from build123d import *

# Parameters (mm, degrees)
BOSS_EXTRUDE1_DEPTH      = 22
BOSS_EXTRUDE1_DEPTH_BACK = 22
SKETCH2_W                = 38
SKETCH2_H                = 20
CUT_EXTRUDE1_DEPTH       = 105.423416914
SKETCH3_W                = 7
SKETCH3_H                = 44
BOSS_EXTRUDE2_DEPTH      = 65.5
SKETCH23_R               = 5
SKETCH23_R_2             = 1.2
CUT_EXTRUDE2_DEPTH       = 111.605436123
SKETCH24_W               = 28.5
SKETCH24_H               = 34
CUT_EXTRUDE3_DEPTH       = 90.954502389
SKETCH26_R               = 1.2
SKETCH26_R_2             = 5
SKETCH26_R_3             = 1.45
CUT_EXTRUDE6_DEPTH       = 107.330263801
SKETCH27_W               = 29.7
SKETCH27_H               = 35.2
CUT_EXTRUDE8_DEPTH       = 73.137455597
SKETCH29_W               = 7
SKETCH29_H               = 30
CUT_EXTRUDE10_DEPTH      = 74.468530678
CHAMFER2_SIZE            = 5


with BuildPart() as part:
    # Sketch1 → Boss-Extrude1 (new, two sides: drawn at the far end of the back side and taken through both)
    with BuildSketch(Plane.XY.offset(-BOSS_EXTRUDE1_DEPTH_BACK)):
        with BuildLine():
            Line((10.25, -60), (10.25, 0))
            ThreePointArc((10.25, 0), (0, -10.25), (-10.25, 0))
            Line((-10.25, 0), (-10.25, -60))
            Line((-10.25, -60), (-10.25, -100))
            Line((-10.25, -100), (10.25, -100))
            Line((10.25, -100), (10.25, -60))
        make_face()
        with BuildLine():
            Line((10.25, 0), (9.2, 0))
            ThreePointArc((9.2, 0), (8.816088231, -0.879772698), (7.91, -1.196620241))
            ThreePointArc((7.91, -1.196620241), (5.656854249, -5.656854249), (1.196620241, -7.91))
            ThreePointArc((1.196620241, -7.91), (1.199154762, -7.954968281), (1.2, -8))
            ThreePointArc((1.2, -8), (-0.045031719, -9.199154762), (-1.196620241, -7.91))
            ThreePointArc((-1.196620241, -7.91), (-5.656854249, -5.656854249), (-7.91, -1.196620241))
            ThreePointArc((-7.91, -1.196620241), (-8.816088231, -0.879772698), (-9.2, 0))
            Line((-9.2, 0), (-10.25, 0))
            ThreePointArc((-10.25, 0), (0, -10.25), (10.25, 0))
        make_face()
        with BuildLine():
            ThreePointArc((7.91, -1.196620241), (7.120227302, -0.816088231), (6.8, 0))
            Line((6.8, 0), (4.2, 0))
            ThreePointArc((4.2, 0), (0, -4.2), (-4.2, 0))
            Line((-4.2, 0), (-6.8, 0))
            ThreePointArc((-6.8, 0), (-7.120227302, -0.816088231), (-7.91, -1.196620241))
            ThreePointArc((-7.91, -1.196620241), (-5.656854249, -5.656854249), (-1.196620241, -7.91))
            ThreePointArc((-1.196620241, -7.91), (0, -6.8), (1.196620241, -7.91))
            ThreePointArc((1.196620241, -7.91), (5.656854249, -5.656854249), (7.91, -1.196620241))
        make_face()
        with BuildLine():
            Line((4.2, 0), (6.8, 0))
            ThreePointArc((6.8, 0), (7.120227302, 0.816088231), (7.91, 1.196620241))
            ThreePointArc((7.91, 1.196620241), (5.656854249, 5.656854249), (1.196620241, 7.91))
            ThreePointArc((1.196620241, 7.91), (0, 6.8), (-1.196620241, 7.91))
            ThreePointArc((-1.196620241, 7.91), (-5.656854249, 5.656854249), (-7.91, 1.196620241))
            ThreePointArc((-7.91, 1.196620241), (-7.120227302, 0.816088231), (-6.8, 0))
            Line((-6.8, 0), (-4.2, 0))
            ThreePointArc((-4.2, 0), (0, 4.2), (4.2, 0))
        make_face()
        with BuildLine():
            ThreePointArc((7.91, 1.196620241), (8.816088231, 0.879772698), (9.2, 0))
            Line((9.2, 0), (10.25, 0))
            ThreePointArc((10.25, 0), (0, 10.25), (-10.25, 0))
            Line((-10.25, 0), (-9.2, 0))
            ThreePointArc((-9.2, 0), (-8.816088231, 0.879772698), (-7.91, 1.196620241))
            ThreePointArc((-7.91, 1.196620241), (-5.656854249, 5.656854249), (-1.196620241, 7.91))
            ThreePointArc((-1.196620241, 7.91), (-0.045031719, 9.199154762), (1.2, 8))
            ThreePointArc((1.2, 8), (1.199154762, 7.954968281), (1.196620241, 7.91))
            ThreePointArc((1.196620241, 7.91), (5.656854249, 5.656854249), (7.91, 1.196620241))
        make_face()
    extrude(amount=BOSS_EXTRUDE1_DEPTH + BOSS_EXTRUDE1_DEPTH_BACK)

    # Sketch2 → Cut-Extrude1 (cut, through all)
    with BuildSketch(Plane.ZY.offset(10.25)):
        with Locations((0, 0.25)):
            Rectangle(SKETCH2_W, SKETCH2_H)
    extrude(amount=-CUT_EXTRUDE1_DEPTH, mode=Mode.SUBTRACT)

    # Sketch3 → Boss-Extrude2 (add)
    with BuildSketch(Plane(origin=(0, -9.75, 0), x_dir=(1, 0, 0), z_dir=(0, 1, 0))):
        with Locations((-13.75, 0)):
            Rectangle(SKETCH3_W, SKETCH3_H)
        with Locations((13.75, 0)):
            Rectangle(SKETCH3_W, SKETCH3_H)
    extrude(amount=-BOSS_EXTRUDE2_DEPTH)

    # Sketch23 → Cut-Extrude2 (cut, through all)
    with BuildSketch(Plane.XY.offset(22)):
        with BuildLine():
            Line((-10.25, -100), (10.25, -100))
            Line((10.25, -100), (10.25, -85))
            ThreePointArc((10.25, -85), (0, -95.25), (-10.25, -85))
            Line((-10.25, -85), (-10.25, -100))
        make_face()
        with Locations((0, -85)):
            Circle(SKETCH23_R)
        with Locations((8, -85)):
            Circle(SKETCH23_R_2)
        with Locations((0, -77)):
            Circle(SKETCH23_R_2)
        with Locations((0, -93)):
            Circle(SKETCH23_R_2)
        with Locations((-8, -85)):
            Circle(SKETCH23_R_2)
    extrude(amount=-CUT_EXTRUDE2_DEPTH, mode=Mode.SUBTRACT)

    # Sketch24 → Cut-Extrude3 (cut, through all)
    with BuildSketch(Plane(origin=(0, -9.75, 0), x_dir=(1, 0, 0), z_dir=(0, 1, 0))):
        Rectangle(SKETCH24_W, SKETCH24_H)
    extrude(amount=-CUT_EXTRUDE3_DEPTH, mode=Mode.SUBTRACT)

    # Sketch26 → Cut-Extrude6 (cut, through all)
    # profile 1 of 5: a face of its own
    with BuildSketch(Plane.XY.offset(22)):
        with BuildLine():
            Line((10.25, -75.25), (14.25, -75.25))
            Line((14.25, -75.25), (14.25, -56.53282359))
            Line((14.25, -56.53282359), (14.25, -56.25))
            Line((14.25, -56.25), (-14.25, -56.25))
            Line((-14.25, -56.25), (-14.25, -56.53282359))
            Line((-14.25, -56.53282359), (-14.25, -75.25))
            Line((-14.25, -75.25), (-10.25, -75.25))
            Line((-10.25, -75.25), (-10.25, -85))
            ThreePointArc((-10.25, -85), (0, -95.25), (10.25, -85))
            Line((10.25, -85), (10.25, -75.25))
        make_face()
        with Locations((-8, -85)):
            Circle(SKETCH26_R, mode=Mode.SUBTRACT)
        with Locations((0, -85)):
            Circle(SKETCH26_R_2, mode=Mode.SUBTRACT)
        with Locations((0, -77)):
            Circle(SKETCH26_R, mode=Mode.SUBTRACT)
        with Locations((0, -93)):
            Circle(SKETCH26_R, mode=Mode.SUBTRACT)
        with Locations((8, -85)):
            Circle(SKETCH26_R, mode=Mode.SUBTRACT)
    # profile 2 of 5: a face of its own
    with BuildSketch(Plane.XY.offset(22)):
        Polygon((-17.25, -75.25), (-14.25, -75.25), (-14.25, -56.53282359), (-14.25, -56.25), (-17.25, -56.25), align=None)
    # profile 3 of 5: a face of its own
    with BuildSketch(Plane.XY.offset(22)):
        Polygon((14.25, -56.53282359), (14.25, -75.25), (17.25, -75.25), (17.25, -56.25), (14.25, -56.25), align=None)
    # profile 4 of 5: a face of its own
    with BuildSketch(Plane.XY.offset(22)):
        with Locations((-11, -53)):
            Circle(SKETCH26_R_3)
    # profile 5 of 5: a face of its own
    with BuildSketch(Plane.XY.offset(22)):
        with Locations((11, -53)):
            Circle(SKETCH26_R_3)
    extrude(amount=-CUT_EXTRUDE6_DEPTH, mode=Mode.SUBTRACT)

    # Sketch27 → Cut-Extrude8 (cut, through all)
    with BuildSketch(Plane.XZ.offset(56.25)):
        Rectangle(SKETCH27_W, SKETCH27_H)
    extrude(amount=-CUT_EXTRUDE8_DEPTH, mode=Mode.SUBTRACT)

    # Sketch29 → Cut-Extrude10 (cut, through all)
    with BuildSketch(Plane(origin=(0, 0, -22), x_dir=(-1, 0, 0), z_dir=(0, 0, -1))):
        with Locations((-13.75, -24.75)):
            Rectangle(SKETCH29_W, SKETCH29_H)
    extrude(amount=-CUT_EXTRUDE10_DEPTH, mode=Mode.SUBTRACT)

    # Chamfer2
    # the kernel refuses this chamfer: 5 mm, written as the material it takes off along each edge
    with BuildSketch(Plane(origin=(-17.25, -56.25, 34.85841494), x_dir=(0.9996219169112968, -0.027495876610586327, 0), z_dir=(0, 0, -1))) as chamfer2_piece_1:
        Polygon((CHAMFER2_SIZE * 0.999621916911, -CHAMFER2_SIZE * 0.0274958766106), (-CHAMFER2_SIZE * 0.0274958766106, -CHAMFER2_SIZE * 0.999621916911), (0, 0), align=None)
    extrude(amount=69.71682988, mode=Mode.SUBTRACT)


solid = part.part
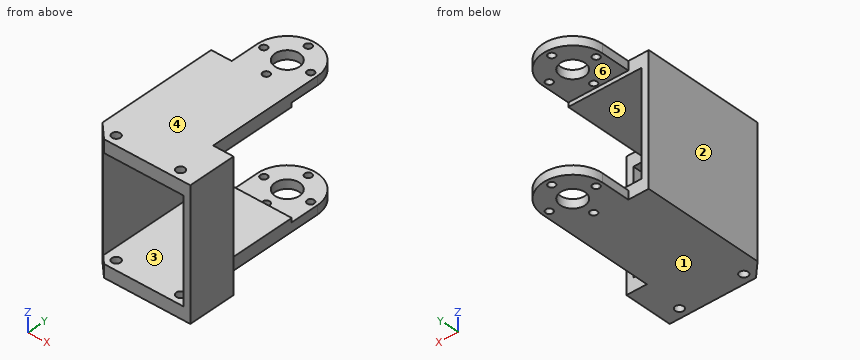
Part model, mm, in its own coordinate system. Face numbers are marked on the shaded views. A direction names the side the tool comes from. Round coordinates to 2 decimals unless told otherwise and drop trailing zeros. Write each loop counter-clockwise with the first axis right and the second up, starting at its lowest first coordinate (ties: lowest second). Pieces come first, ordered by that corner, then holes. Notation, with made-up numbers: M 57,-33 L 90,-33 A20 ccw 90,-1 Z; hole C 89,81.5 d3. An arc over 180 degrees is marked long. Return JSON: item names as keys, results as strings. Group by question number.
(1) Saw through at A-A on x = -11. Write the cut outline in (y, z).
(2) Drill centre lines: probe 1 along Z at (x, y) = (0.5, -19); probe 2 along Z at (x, y) = (-6, -6); probe 3 along Y at (x, z) = (-11, -18.8). Where is each one in solid material? Low to high.
(3) Which spindle directions (+Z, -Z, +X, -X, +Y, -Y) get a long thin tool onto all of the face, cutting with end or side? Do the marked faces 4, 5 and 6. Say none if no direction does.
(4) Two-plate mould, pull along X, no slides. Class the marked faces 1, 2 and 3: +X half, -X half, draft (parallel to the pull), parting line (faces both ways), or undercut.
(5) Saw through at C-C on z = -13. Write the cut outline in (x, y).
(6) Pin check, flat tips, straight feed: pin 1 Ø1.3 at (y, z) = (-28, 20.5) entering from +X; pin 2 Ø1.7 at (x, y) = (-11, -53) entering from +Z; pin 3 Ø4 at (y, z) = (-12.5, 14) entering from +X. Stop position of each tip, or through.
(7) Saw through at D-D on y = -38. Write the cut outline in (x, z).
(8) Saw through at B-B on y = -48. Write the cut outline in (x, z).
Returned:
{
 "1": {"outline": "M -56.25,-22 L -54.45,-22 L -54.45,-17.6 L -56.25,-17.6 Z; M -56.25,17.6 L -54.45,17.6 L -54.45,22 L -56.25,22 Z; M -51.55,-22 L -9.75,-22 L -9.75,-17.6 L -51.55,-17.6 Z; M -51.55,17.6 L -9.75,17.6 L -9.75,22 L -51.55,22 Z"},
 "2": {"probe 1": "-22 to -17.6, 17.6 to 22", "probe 2": "-22 to -19, 19 to 22", "probe 3": "-56.25 to -54.45, -51.55 to -9.75"},
 "3": {"face 4": "+Z, +X, -X, +Y, -Y", "face 5": "+Y, -Y", "face 6": "+X, -X, +Y"},
 "4": {"face 1": "draft", "face 2": "-X half", "face 3": "undercut"},
 "5": {"outline": "M -17.25,-51.25 L -14.85,-53.65 L -14.85,-9.75 L -17.25,-9.75 Z; M 14.85,-56.25 L 17.25,-56.25 L 17.25,-39.75 L 14.85,-39.75 Z"},
 "6": {"pin 1": "x = 10.25", "pin 2": "through", "pin 3": "x = -14.85"},
 "7": {"outline": "M -17.25,-22 L 10.25,-22 L 10.25,-17.6 L -14.85,-17.6 L -14.85,17.6 L 10.25,17.6 L 10.25,22 L -17.25,22 Z"},
 "8": {"outline": "M -17.25,-22 L 17.25,-22 L 17.25,22 L -17.25,22 Z; hole M -14.85,-17.6 L 14.85,-17.6 L 14.85,17.6 L -14.85,17.6 Z"}
}
